Can you work these out from the model? Positions are in its coordinate system, mm. Face numbers are marked on the shaded views. A direction names the side the tool comes from. Coordinates: 2 decimals unless noted, no trailing zeros. Order: outer loops, then holes, each group sorted by start corner. A loop starts at its lowest first (then second) coordinate and runs counter-clockwise, first axis right, second up. Notation, with made-up numbers: (77.25, 54.5) -> (99.25, 54.5) arc R19 cw to (99.25, 77.5) -> close; hole circle Ø8 at (-13.75, 61.5). An arc over 180 degrees is marked (long way). Write item = value, one per line.
```python
from build123d import *

# Parameters (mm, degrees)
SKETCH1_W           = 20
SKETCH1_H           = 18
BOSS_EXTRUDE1_DEPTH = 35
CHAMFER1_SIZE       = 2
SKETCH4_W           = 2
SKETCH4_H           = 1
CUT_EXTRUDE2_DEPTH  = 19
BOSS_EXTRUDE3_START = -2
BOSS_EXTRUDE3_DEPTH = 12
SKETCH2_R           = 4
CUT_EXTRUDE1_DEPTH  = 35
SKETCH8_R           = 4
SKETCH9_R           = 4
BOSS_EXTRUDE4_START = -6
SKETCH10_W          = 19.5
SKETCH10_H          = 13.5
SKETCH10_R          = 5
BOSS_EXTRUDE4_DEPTH = 1
LPATTERN1_COUNT     = 3
LPATTERN1_PITCH     = 1.5
BOSS_EXTRUDE5_DEPTH = 0.75


with BuildPart() as part:
    # Sketch1 → Boss-Extrude1 (new body)
    with BuildSketch(Plane.XY):
        Rectangle(SKETCH1_W, SKETCH1_H)
    extrude(amount=BOSS_EXTRUDE1_DEPTH)

    # Chamfer1
    chamfer1_edges = [part.edges().sort_by_distance(p)[0] for p in [
        (10, 9, 17.5),
        (10, -9, 17.5),
        (-10, -9, 17.5),
        (-10, 9, 17.5),
    ]]
    chamfer(chamfer1_edges, length=CHAMFER1_SIZE)

    # Sketch4 → Cut-Extrude2 (cut, through all)
    with BuildSketch(Plane.XZ.offset(9)):
        with Locations((-9, 10)):
            Rectangle(SKETCH4_W, SKETCH4_H)
        with Locations((-9, 11.75)):
            Rectangle(SKETCH4_W, SKETCH4_H)
        with Locations((-9, 13.5)):
            Rectangle(SKETCH4_W, SKETCH4_H)
        with Locations((-9, 15.25)):
            Rectangle(SKETCH4_W, SKETCH4_H)
        with Locations((-9, 17)):
            Rectangle(SKETCH4_W, SKETCH4_H)
        with Locations((9, 17)):
            Rectangle(SKETCH4_W, SKETCH4_H)
        with Locations((9, 15.25)):
            Rectangle(SKETCH4_W, SKETCH4_H)
        with Locations((9, 13.5)):
            Rectangle(SKETCH4_W, SKETCH4_H)
        with Locations((9, 11.75)):
            Rectangle(SKETCH4_W, SKETCH4_H)
        with Locations((9, 10)):
            Rectangle(SKETCH4_W, SKETCH4_H)
    extrude(amount=-CUT_EXTRUDE2_DEPTH, mode=Mode.SUBTRACT)

    # Sketch7 → Boss-Extrude3 (add)
    with BuildSketch(Plane.XZ.offset(9).offset(BOSS_EXTRUDE3_START)):
        Polygon((-8.923003752, 2.34947146), (8.923003752, 0), (7.61774183, -9.914448614), (-10.228265675, -7.564977154), align=None)
    extrude(amount=-BOSS_EXTRUDE3_DEPTH)

    # Sketch2 → Cut-Extrude1 (cut)
    with BuildSketch(Plane.XY.offset(35)):
        with Locations((0, -1)):
            Circle(SKETCH2_R)
    extrude(amount=-CUT_EXTRUDE1_DEPTH, mode=Mode.SUBTRACT)

    # Sketch8 → Cut-Loft1 section 0
    with BuildSketch(Plane(origin=(-1.153239932, 0, -8.759726958), x_dir=(-0.991444861, 0, 0.130526192), z_dir=(-0.130526192, 0, -0.991444861))):
        with Locations((0, -1)):
            Circle(SKETCH8_R)
    # Sketch9 → Cut-Loft1 section 1
    with BuildSketch(Plane.XY):
        with Locations((0, -1)):
            Circle(SKETCH9_R)
    loft(mode=Mode.SUBTRACT)

    # Sketch10 → Boss-Extrude4 (add)
    with BuildSketch(Plane(origin=(-1.153239932, 0, -8.759726958), x_dir=(-0.991444861, 0, 0.130526192), z_dir=(-0.130526192, 0, -0.991444861)).offset(BOSS_EXTRUDE4_START)):
        with Locations((0.153333782, -1)):
            Rectangle(SKETCH10_W, SKETCH10_H)
        with Locations((0, -1)):
            Circle(SKETCH10_R, mode=Mode.SUBTRACT)
    boss_extrude4 = extrude(amount=-BOSS_EXTRUDE4_DEPTH)

    # LPattern1: Boss-Extrude4 ×3
    with Locations(*[Vector(-0.130526192, 0, -0.991444861) * (i * LPATTERN1_PITCH) for i in range(1, LPATTERN1_COUNT)]):
        add(boss_extrude4)

    # Sketch11 → Boss-Extrude5 (add)
    with BuildSketch(Plane.XZ.offset(7)):
        Polygon((-9.706160906, -3.599197708), (8.139846599, -5.948669168), (8.400898983, -3.965779445), (-9.445108521, -1.616307986), align=None)
    extrude(amount=BOSS_EXTRUDE5_DEPTH)


solid = part.part
```
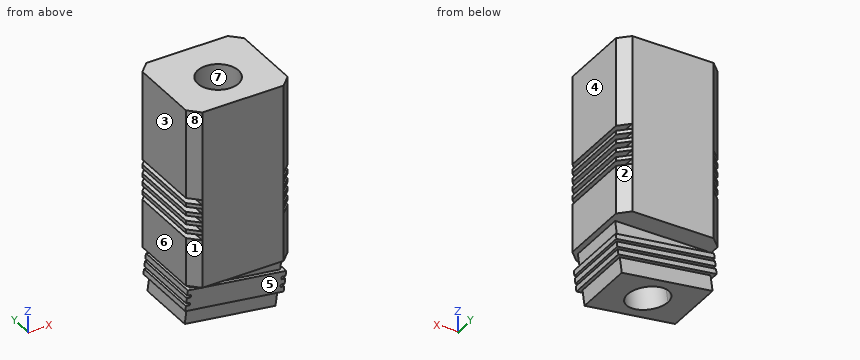
Item 1: If I drill on probe 1 along Z at (x, y) = (-9.5, 7.25); probe 2 along Y at (x, z) = (0, 7.5); probe 3 along X at (y, z) = (3.5, 0.5), over which ranges is the centre line in solid material (lowest first)?
A:
probe_1 = 0 to 9.5, 10.5 to 11.25, 12.25 to 13, 14 to 14.75, 15.75 to 16.5, 17.5 to 35
probe_2 = -9 to -5, 3 to 9
probe_3 = -10 to 10
Item 2: If we mould it in two halves opening along Y, with no side actions, what happens to the marked faces 6, 7 and 8? For each: pulls with the +Y half, pulls with the -Y half, needs draft (parallel to the pull), parting line crosses it, or undercut.
A:
face_6 = needs draft
face_7 = undercut
face_8 = pulls with the -Y half
Item 3: I'm going to push flat-ended pins straight in: P1, Ø1.5, axis at y = -4.5, z = 15, coming from the -X side; P2, Ø4, axis at x = 3.5, z = -2.5, coming from the +Y side; P3, Ø0.8, axis at y = -2.5, z = 10, coming from the -X side. Where does each tip first touch, or does it pass through?
A:
P1 = -10
P2 = 5.75
P3 = -8
Item 4: For the marked faces 1, 2, 3, 4 and 5, which set-ups out of +Z, -Z, +X, -X, +Y, -Y let a thin tool reach every point of the face, with its end or its side?
A:
face_1 = +Z, -X, -Y
face_2 = +Z, -Z, +X, +Y
face_3 = +Z, -X, +Y, -Y
face_4 = +Z, -Z, +X, +Y, -Y
face_5 = -Z, +X, -X, -Y
Item 5: I want a section at B-B, the plane x = -8.5. Give the number of separate pieces and of enclosed holes in the cut face, plus the area to 3 significant figures.
A:
separate_pieces = 6
enclosed_holes = 0
area = 609 mm2
Item 6: I want a section at A-A, the plane z = 6. Please give me the cut outline in (x, y), plus the area to 3 significant figures.
A:
outline = (-10, -7) -> (-8, -9) -> (8, -9) -> (10, -7) -> (10, 7) -> (8, 9) -> (-8, 9) -> (-10, 7) -> close; hole circle Ø8 at (0, -1)
area = 302 mm2
Item 7: I want a section at C-C, the plane x = 6.75. Please give me the cut outline in (y, z), plus the area to 3 significant figures.
A:
outline = (-9, 0) -> (-7, 0) -> (-7, -2.74) -> (-7.75, -2.74) -> (-7.75, -6.77) -> (-7, -6.77) -> (-7, -9.8) -> (5, -9.8) -> (5, -6.77) -> (5.75, -6.77) -> (5.75, -5.77) -> (5, -5.77) -> (5, -5.26) -> (5.75, -5.26) -> (5.75, -4.25) -> (5, -4.25) -> (5, -3.75) -> (5.75, -3.75) -> (5.75, -2.74) -> (5, -2.74) -> (5, 0) -> (9, 0) -> (9, 35) -> (-9, 35) -> close
area = 753 mm2
